from build123d import *

# Parameters (mm, degrees)
SKETCH_1_R           = 37.5
EXTRUDE_1_DEPTH      = 31
SKETCH_2_R           = 31.5
EXTRUDE_2_DEPTH      = 6.5
SKETCH_3_R           = 15.75
CUT_EXTRUDE_1_DEPTH  = 6.5
SKETCH_4_R           = 15.8
EXTRUDE_3_DEPTH      = 6.2
HOLE_WIZARD_M6_1_D   = 5
MM_1_D               = 6
MM_1_DEPTH           = 6
MM_1_TIP             = 1.802581857
EXTRUDE_4_REACH      = 116.985
EXTRUDE_4_END_RADIUS = 37.5
SKETCH_16_R          = 3.457756213
FILLET_2_R           = 1


with BuildPart() as part:
    # 草图1 → 凸台-拉伸1 (new body)
    with BuildSketch(Plane(origin=(0, 0, 0), x_dir=(1, 0, 0), z_dir=(0, 1, 0))):
        with Locations(Location((0, 0, 0), (0, 0, 270))):
            Circle(SKETCH_1_R)
    extrude(amount=EXTRUDE_1_DEPTH)

    # 草图2 → 凸台-拉伸2 (add)
    with BuildSketch(Plane(origin=(0, 31, 0), x_dir=(1, 0, 0), z_dir=(0, 1, 0))):
        with Locations(Location((0, 0, 0), (0, 0, 90))):
            Circle(SKETCH_2_R)
    extrude(amount=EXTRUDE_2_DEPTH)

    # 草图3 → 切除-拉伸1 (cut)
    with BuildSketch(Plane(origin=(0, 37.5, 0), x_dir=(1, 0, 0), z_dir=(0, 1, 0))):
        with Locations(Location((0, 0, 0), (0, 0, 270))):
            Circle(SKETCH_3_R)
    extrude(amount=-CUT_EXTRUDE_1_DEPTH, mode=Mode.SUBTRACT)

    # 草图4 → 凸台-拉伸3 (add)
    with BuildSketch(Plane.XZ):
        with Locations(Location((0, 0, 0), (0, 0, 90))):
            Circle(SKETCH_4_R)
    extrude(amount=EXTRUDE_3_DEPTH)

    # M6 螺纹孔1 (through all)
    with Locations(Plane(origin=(0, 37.5, 0), x_dir=(1, 0, 0), z_dir=(0, 1, 0))):
        with Locations((-23.818134331, -9.107495647), (9.107495647, -23.818134331), (23.818134331, 9.107495647), (-9.107495647, 23.818134331)):
            Hole(HOLE_WIZARD_M6_1_D / 2)

    # 大小mm 暗销孔1
    with Locations(Plane(origin=(0, 37.5, 0), x_dir=(1, 0, 0), z_dir=(0, 1, 0))):
        with Locations((-23.281936233, 10.401992369)):
            Hole(MM_1_D / 2, depth=MM_1_DEPTH)
            with Locations((0, 0, -(MM_1_DEPTH + MM_1_TIP / 2))):  # 118° drill point
                Cone(0, MM_1_D / 2, MM_1_TIP, mode=Mode.SUBTRACT)

    # 凸台-拉伸4: up to this cylinder (the profile starts outside it)
    extrude_4_end = Plane(origin=(0, 17.698511, 0), z_dir=(0, -1, 0)) * Cylinder(EXTRUDE_4_END_RADIUS, 309.97, mode=Mode.PRIVATE)
    # 草图16 → 凸台-拉伸4 (add, up to the surface)
    with BuildSketch(Plane(origin=(52.498483662, 0, 23.455472989), x_dir=(0.4079212693781409, 0, -0.9130171071721089), z_dir=(0.9130171071721089, 0, 0.4079212693781409)), mode=Mode.PRIVATE) as extrude_4_sk1:
        with Locations((0, 17.698511035)):
            Circle(SKETCH_16_R)
    extrude_4_tool1 = extrude(extrude_4_sk1.sketch, amount=-EXTRUDE_4_REACH, mode=Mode.PRIVATE) - extrude_4_end
    add(extrude_4_tool1.solids().sort_by_distance((52.498484, 17.698511, 23.455473))[0])

    # 圆角2
    fillet_2_edges = [part.edges().sort_by_distance(p)[0] for p in [
        (0, 37.5, -15.75),
        (0, 0, -37.5),
        (0, 31, -37.5),
        (0, 37.5, 31.5),
    ]]
    fillet(fillet_2_edges, radius=FILLET_2_R)


solid = part.part
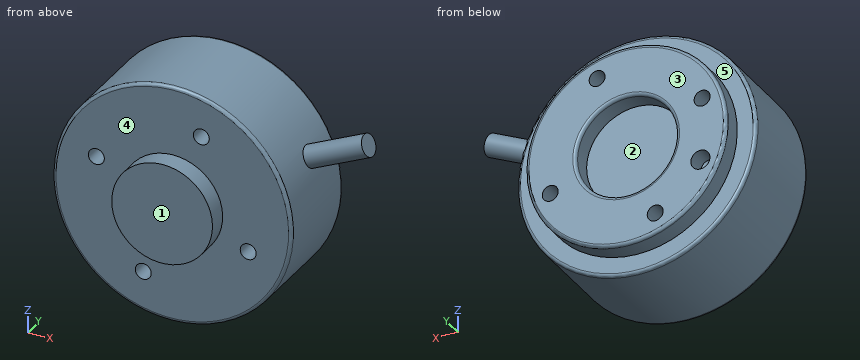
Read the model definition and answer for the solid it produces. Units are mm, in the model's axes. Face numbers are marked on the shaded views. A direction names the side the tool comes from. Give positions to 0.01 mm unless a question says otherwise; leave off trailing zeros. Write each loop counter-clockwise with the first axis right and the second up, starting at its lowest first coordinate (ties: lowest second). Pieces come first, ordered by that corner, then holes. Notation, with made-up numbers: (82.5, 49.25) - (106.5, 49.25) arc R32 cw to (106.5, 83.25) - close; hole circle Ø3 at (12, 51.5). An arc over 180 degrees is marked (long way). Use CSV: the item, a comma, the result in double quotes. Start each with the question number.
(1) Determine the mould class of the marked faces 1 and 2 for opening direction X: +X half, -X half, draft (parallel to the pull), parting line (faces both ways), or undercut.
(2) Given P1, Ø1, axis at y = 11, z = 6.5, coming from the -X side; P2, Ø1.5, axis at x = 10, y = -1.5, coming from the -Z side; P3, Ø10, axis at x = 24, y = 12.5, coming from the +Z side, each flat-ended and moving along its own axis, determine where each tip first touches the part or whether it passes through.
(3) Find section C-C (y = -1.5). Give the vertices of the cut face in (x, z), plus the area to 3 significant figures.
(4) For the marked faces 3, 4 and 5, determine the directions among +Z, -Z, +X, -X, +Y, -Y from which every point of the face is accessible in a straight line to the end or side of a thin tool.
(5) Find section B-B (x = 0). Give the vertices of the cut face in (y, z), plus the area to 3 significant figures.
(6) Consider line 1 along Y through (x, z) = (16, -18.5); line 2 along Y through (x, z) = (15.5, -2.5); line 3 along X through (y, z) = (30, 22.5). Determine where each line is inside the solid, lowest interval first.
(7) Find section A-A (z = 0). Give the vertices of the cut face in (x, y), plus the area to 3 significant figures.
Findings below:
1,face 1,"draft"
1,face 2,"undercut"
2,P1,"x = -37.02"
2,P2,"z = -12.81"
2,P3,"z = 32.33"
3,outline,"circle Ø31.6 at (0, 0)"
3,area,"784 mm2"
4,face 3,"+Z, -Z, +X, -X, +Y"
4,face 4,"-Y"
4,face 5,"+Y"
5,outline,"(-6.2, -15.8) - (0, -15.8) - (0, -36.5) arc R1 ccw to (1, -37.5) - (30, -37.5) arc R1 ccw to (31, -36.5) - (31, -31.5) - (36.5, -31.5) arc R1 ccw to (37.5, -30.5) - (37.5, -16.75) arc R1 ccw to (36.5, -15.75) - (31, -15.75) - (31, 15.75) - (36.5, 15.75) arc R1 ccw to (37.5, 16.75) - (37.5, 30.5) arc R1 ccw to (36.5, 31.5) - (31, 31.5) - (31, 36.5) arc R1 ccw to (30, 37.5) - (1, 37.5) arc R1 ccw to (0, 36.5) - (0, 15.8) - (-6.2, 15.8) - close"
5,area,"2,720 mm2"
6,line 1,"0 to 37.5"
6,line 2,"-6.2 to 31"
6,line 3,"-30 to 6.98, 11.23 to 30"
7,outline,"(-37.5, 1) arc R1 ccw to (-36.5, 0) - (-15.8, 0) - (-15.8, -6.2) - (15.8, -6.2) - (15.8, 0) - (36.5, 0) arc R1 ccw to (37.5, 1) - (37.5, 30) arc R1 ccw to (36.5, 31) - (31.5, 31) - (31.5, 36.5) arc R1 ccw to (30.5, 37.5) - (16.75, 37.5) arc R1 ccw to (15.75, 36.5) - (15.75, 31) - (-15.75, 31) - (-15.75, 36.5) arc R1 ccw to (-16.75, 37.5) - (-30.5, 37.5) arc R1 ccw to (-31.5, 36.5) - (-31.5, 31) - (-36.5, 31) arc R1 ccw to (-37.5, 30) - close"
7,area,"2,720 mm2"
